Input: part model. Units: mm. Frame: model coordinates. A direction names the side the tool comes from. Give positions to 0.01 mm unless a question says otherwise; leave off trailing zeros. Order: outer loops, then holes, each group sorted by start corner. A loop starts at its lowest first (then second) coordinate and runs counter-clockwise, first axis right, second up. Notation, with made-up numbers: (-25.5, 70.25) - (17.5, 70.25) arc R18 cw to (17.5, 84.25) - close; hole circle Ø6 at (85, -18.5). An arc over 180 degrees is marked (long way). Use a Markdown table: item, result.
from build123d import *

# Parameters (mm, degrees)
F0_W     = 31.75
F0_H     = 88.9
F0_H_2   = 31.75
F0_R     = 15.875
F1_DEPTH = 31.75
F2_DEPTH = 73.025
F3_DEPTH = 73.025
F4_DEPTH = 92.075
F5_DEPTH = 53.975


# Not quite as in the source:
# - a feature names something its author has since deleted; it is built from what else it names


with BuildPart() as f1:
    # F0 (on Front) → F1 (new body)
    with BuildSketch(Plane.XZ):
        Polygon((114.6503422856, 101.6), (57.5003422856, 101.6), (57.5003422856, 69.85), (57.5003422856, -19.05), (57.5003422856, -50.8), (114.6503422856, -50.8), (114.6503422856, 0), (73.3753422856, 0), (73.3753422856, 50.8), (114.6503422856, 50.8), align=None)
        with Locations((41.6253422856, 25.4)):
            Rectangle(F0_W, F0_H)
        with Locations((41.6253422856, -34.925)):
            Rectangle(F0_W, F0_H_2)
        Polygon((-12.3496577144, 101.6), (-50.4496577144, 101.6), (-50.4496577144, 69.85), (-50.4496577144, -19.05), (-50.4496577144, -50.8), (25.7503422856, -50.8), (25.7503422856, -19.05), (25.7503422856, 69.85), (25.7503422856, 101.6), align=None)
        with Locations((-12.3496577144, 25.4)):
            Circle(F0_R, mode=Mode.SUBTRACT)
        with Locations((-66.3246577144, 25.4)):
            Rectangle(F0_W, F0_H)
        with Locations((-66.3246577144, -34.925)):
            Rectangle(F0_W, F0_H_2)
        with Locations((-66.3246577144, 85.725)):
            Rectangle(F0_W, F0_H_2)
        with Locations((41.6253422856, 85.725)):
            Rectangle(F0_W, F0_H_2)
    extrude(amount=F1_DEPTH)

    # F0 (on Front) → F2 (join)
    with BuildSketch(Plane.XZ):
        with Locations((-66.3246577144, 25.4)):
            Rectangle(F0_W, F0_H)
        with Locations((-66.3246577144, -34.925)):
            Rectangle(F0_W, F0_H_2)
    extrude(amount=F2_DEPTH)

    # F0 (on Front) → F3 (join)
    with BuildSketch(Plane.XZ):
        with Locations((41.6253422856, -34.925)):
            Rectangle(F0_W, F0_H_2)
        with Locations((41.6253422856, 25.4)):
            Rectangle(F0_W, F0_H)
    extrude(amount=F3_DEPTH)

    # F0 (on Front) → F4 (join)
    with BuildSketch(Plane.XZ):
        with Locations((-66.3246577144, -34.925)):
            Rectangle(F0_W, F0_H_2)
        with Locations((41.6253422856, -34.925)):
            Rectangle(F0_W, F0_H_2)
    extrude(amount=F4_DEPTH)

    # F0 (on Front) → F5 (join)
    with BuildSketch(Plane.XZ):
        Polygon((-12.3496577144, 101.6), (-50.4496577144, 101.6), (-50.4496577144, 69.85), (-50.4496577144, -19.05), (-50.4496577144, -50.8), (25.7503422856, -50.8), (25.7503422856, -19.05), (25.7503422856, 69.85), (25.7503422856, 101.6), align=None)
        with Locations((-12.3496577144, 25.4)):
            Circle(F0_R, mode=Mode.SUBTRACT)
    extrude(amount=F5_DEPTH)


solid = f1.part
1. Section query A-A (y = -9.5). Return loops of the section in (x, z) (3 decimals), then the cut area to 3 significant figures.
Response:
| item | result |
|---|---|
| outline | (-82.2, -50.8) - (114.65, -50.8) - (114.65, 0) - (73.375, 0) - (73.375, 50.8) - (114.65, 50.8) - (114.65, 101.6) - (-82.2, 101.6) - close; hole circle Ø31.75 at (-12.35, 25.4) |
| area | 27,100 mm^2 |
2. Pin query (flat end, axial travel): pin 1 (18 mm diameter, centred on y = -41, z = 91, fed in from +X); pin 2 (9.5 mm diameter, centred on x = 41, z = 47.5, fed in from -Y) (3 decimals); pin 3 (16 mm diameter, centred on x = -67, y = -55, fed in from +Z). Return the tip coordinate at first contact, or that it passes through.
Response:
| item | result |
|---|---|
| pin 1 | stops at x = 25.75 |
| pin 2 | stops at y = -73.025 |
| pin 3 | stops at z = 69.85 |
3. Set-up query: faces 1 (the face through (25.75, -43, 86)), 2 (the face through (-67, -52, 69.85)), 3 (the face through (41, -82, -19.05)), 4 (the face through (-50.45, -69, -5)), 5 (the face through (94, -16, 50.8)). Return all of +Z, -Z, +X, -X, +Y, -Y with unobstructed straight access to the full face (end or side cutting, diameter ignored); none if empty.
Response:
| item | result |
|---|---|
| face 1 | +Z, +X, -Y |
| face 2 | +Z, -X, -Y |
| face 3 | +Z, +X, -X, -Y |
| face 4 | +Z, -Z, -Y |
| face 5 | +X, +Y, -Y |
4. Section query B-B (z = 25.4). Return loops of the section in (x, y) (3 decimals).
Response:
| item | result |
|---|---|
| outline | (-82.2, -73.025) - (-50.45, -73.025) - (-50.45, -53.975) - (-28.225, -53.975) - (-28.225, 0) - (-82.2, 0) - close; (3.525, -53.975) - (25.75, -53.975) - (25.75, -73.025) - (57.5, -73.025) - (57.5, -31.75) - (73.375, -31.75) - (73.375, 0) - (3.525, 0) - close |
5. Section query C-C (x = 80). Return loops of the section in (y, z), then the cut area to 3 significant figures.
Response:
| item | result |
|---|---|
| outline | (-31.75, -50.8) - (0, -50.8) - (0, 0) - (-31.75, 0) - close; (-31.75, 50.8) - (0, 50.8) - (0, 101.6) - (-31.75, 101.6) - close |
| area | 3,230 mm^2 |
6. Section query D-D (y = -58). Return loops of the section in (x, z).
Response:
| item | result |
|---|---|
| outline | (-82.2, -50.8) - (-50.45, -50.8) - (-50.45, 69.85) - (-82.2, 69.85) - close; (25.75, -50.8) - (57.5, -50.8) - (57.5, 69.85) - (25.75, 69.85) - close |
7. Material intervals for line 1 along X through (y, z) = (-30, 25); line 2 along X through (y, z) = (-34, 25); line 3 along Z through (x, y) = (78, -15.5), sorted ascending.
Response:
| item | result |
|---|---|
| line 1 | x = -82.2 to -28.22, 3.52 to 73.38 |
| line 2 | x = -82.2 to -28.22, 3.52 to 57.5 |
| line 3 | z = -50.8 to 0, 50.8 to 101.6 |
8. Mould query, pull axis Z, two halves, no side actions, for faces 6 (the face through (41, -52, 69.85)), 7 (the face through (-3.82, -26.61, 38.79)), 8 (the face through (73.375, -16, 25)), 9 (the face through (-50.45, -43, 86)). Classes: pulls with the +Z half, pulls with the -Z half, needs draft (parallel to the pull), parting line crosses it, or undercut.
Response:
| item | result |
|---|---|
| face 6 | pulls with the +Z half |
| face 7 | undercut |
| face 8 | undercut |
| face 9 | needs draft |
